Verification items for the finished model (mm, model axes). A direction names the side the tool comes from. Round coordinates to 2 decimals unless told otherwise and drop trailing zeros. Order: outer loops, then holes, each group sorted by start corner. A loop starts at its lowest first (then second) coordinate and runs counter-clockwise, first axis right, second up. Notation, with made-up numbers: M 7,20 L 26,20 A18 ccw 26,37 Z; hole C -8,12 d5. An arc over 180 degrees is marked long. One line per item, written item: value. Start each with the question number.
from build123d import *


with BuildPart() as part:
    # Sketch1 → Revolve1 (revolve)
    with BuildSketch(Plane.XY, mode=Mode.PRIVATE) as revolve1_sk:
        with BuildLine():
            Line((0, 7.3), (0, 5.3))
            ThreePointArc((0, 5.3), (0.087867966, 5.087867966), (0.3, 5))
            Line((0.3, 5), (7.7, 5))
            ThreePointArc((7.7, 5), (7.912132034, 5.087867966), (8, 5.3))
            Line((8, 5.3), (8, 7.3))
            ThreePointArc((8, 7.3), (7.970710678, 7.370710678), (7.9, 7.4))
            Line((7.9, 7.4), (5.849097347, 7.4))
            ThreePointArc((5.849097347, 7.4), (4, 6.519), (2.150902653, 7.4))
            Line((2.150902653, 7.4), (0.1, 7.4))
            ThreePointArc((0.1, 7.4), (0.029289322, 7.370710678), (0, 7.3))
        make_face()
    revolve(revolve1_sk.sketch.rotate(Axis((50, 0, 0), (-1, 0, 0)), 270), axis=Axis((50, 0, 0), (-1, 0, 0)))

    # Sketch2 → Cut-Revolve1 (revolve, cut)
    with BuildSketch(Plane.XY, mode=Mode.PRIVATE) as cut_revolve1_sk:
        with BuildLine():
            Line((0, 9.975), (0, 6.275))
            Line((0, 6.275), (0.285, 6.275))
            ThreePointArc((0.285, 6.275), (0.444099026, 6.340900974), (0.51, 6.5))
            Line((0.51, 6.5), (0.51, 9.525))
            Line((0.51, 9.525), (7.49, 9.525))
            Line((7.49, 9.525), (7.49, 6.5))
            ThreePointArc((7.49, 6.5), (7.555900974, 6.340900974), (7.715, 6.275))
            Line((7.715, 6.275), (8, 6.275))
            Line((8, 6.275), (8, 9.975))
            Line((8, 9.975), (0, 9.975))
        make_face()
    revolve(cut_revolve1_sk.sketch.rotate(Axis((50, 0, 0), (-1, 0, 0)), 270), axis=Axis((50, 0, 0), (-1, 0, 0)), mode=Mode.SUBTRACT)

    # Sketch3 → Revolve2 (revolve)
    with BuildSketch(Plane.XY, mode=Mode.PRIVATE) as revolve2_sk:
        Polygon((0.27, 11.3), (0.315, 10.04375), (0.27, 8.7875), (0.27, 6.275), (0.36, 6.275), (0.45, 8.7875), (0.45, 10.04375), (0.36, 11.3), align=None)
    revolve(revolve2_sk.sketch.rotate(Axis((50, 0, 0), (-1, 0, 0)), 270), axis=Axis((50, 0, 0), (-1, 0, 0)))

    # Sketch4 → Revolve3 (revolve)
    with BuildSketch(Plane.XY, mode=Mode.PRIVATE) as revolve3_sk:
        Polygon((7.55, 10.04375), (7.55, 8.7875), (7.64, 6.275), (7.73, 6.275), (7.73, 8.7875), (7.685, 10.04375), (7.73, 11.3), (7.64, 11.3), align=None)
    revolve(revolve3_sk.sketch.rotate(Axis((50, 0, 0), (-1, 0, 0)), 270), axis=Axis((50, 0, 0), (-1, 0, 0)))


solid = part.part
1. Draft check along Y on faces 1 (the face through (0, -5, -3)), 2 (the face through (4.05, -4.88, -1.08)), 3 (the face through (6.658, -7.224, -1.604)). Enter one of: released by +Y, released by -Y, zero draft, split by the parting line, or undercut.
2. Section check B-B (x = 4.75). Record the cut outline in (y, z).
3. Scan lines: line 1 along Y through (x, z) = (2, 0); line 2 along Z through (x, y) = (1.25, 1.5); line 3 along X through (y, z) = (6.5, 6.75). Record each from-to range of solid material in increasing order.
4. Section check A-A (x = 1.5). Record the cut outline in (y, z).
5. Tool access check on faces 4 (the face through (8, -5, 3)), 5 (the face through (7.55, -9, 0)). Record the directions out of +Z, -Z, +X, -X, +Y, -Y that give a thin tool (end or side, any length) a straight path to the whole face; none if there is none.
6. Depth check by flat-ended pin: pin 1 (13 mm diameter, centred on y = 0, z = 0, fed in from -X); pin 2 (2 mm diameter, centred on x = 3.5, y = 1, fed in from +Z); pin 3 (5 mm diameter, centred on y = 7, z = -7.5, fed in from -X); pin 4 (4 mm diameter, centred on x = 5, z = -6.5, fed in from +Y). Enter the tip coordinate at first touch or a pass-through.
Geometry check:
1. face 1: zero draft
1. face 2: undercut
1. face 3: split by the parting line
2. outline: C 0,0 d13.28; hole C 0,0 d10
3. line 1: y = -7.4 to -5, 5 to 7.4
3. line 2: z = -7.25 to -4.77, 4.77 to 7.25
3. line 3: x = 0.29 to 0.45, 7.55 to 7.71
4. outline: C 0,0 d14.8; hole C 0,0 d10
5. face 4: +Z, -Z, +X, +Y, -Y
5. face 5: none
6. pin 1: stops at x = 0
6. pin 2: stops at z = 6.99
6. pin 3: stops at x = 0.27
6. pin 4: stops at y = 5.72
